from build123d import *

# Parameters (mm, degrees)
F0_W     = 28.575
F0_H     = 52.07
F1_DEPTH = 50.8
F2_R     = 11.1252
F3_DEPTH = 50.801
F4_R     = 1.5875
F5_DEPTH = 25.4


with BuildPart() as f1:
    # F0 (on Front) → F1 (new body)
    with BuildSketch(Plane.XZ):
        Rectangle(F0_W, F0_H)
    extrude(amount=F1_DEPTH)

    # F2 (on face) → F3 (cut, through all)
    with BuildSketch(Plane.XZ.offset(50.8)):
        with Locations((0, 11.641667)):
            Circle(F2_R)
        with Locations((0, -11.641667)):
            Circle(F2_R)
    extrude(amount=-F3_DEPTH, mode=Mode.SUBTRACT)

    # F4 (on face) → F5 (cut)
    with BuildSketch(Plane.YZ.offset(14.2875)):
        with Locations((-19.05, 0)):
            Circle(F4_R)
    extrude(amount=-F5_DEPTH, mode=Mode.SUBTRACT)


solid = f1.part
Work out the finished part from the listing and answer in its coordinate system (mm). A direction names the side the tool comes from. Coordinates: 2 decimals unless noted, no trailing zeros. Loops run counter-clockwise (first coordinate to the right, second up) from the corner with the lowest first, then second, coordinate; pieces in that order, holes last. Notation, with made-up numbers: (-9, 5.5) -> (31, 5.5) arc R18 ccw to (31, 30.5) -> close; hole circle Ø6 at (-19, 65). An arc over 180 degrees is marked (long way). Answer as CSV lines item,"result".
1) For faces 4 (the face through (1.765, -17.536, 0.477)), 5 (the face through (5.981, -25.756, 21.022)), determine the directions among +Z, -Z, +X, -X, +Y, -Y from which every point of the face is accessible in a straight line to the end or side of a thin tool.
A:
face 4,"+X"
face 5,"+Y, -Y"
2) Straight lines are drawn through the part: probe 1 along Z at (x, y) = (0, -23) (3 decimals); probe 2 along Z at (x, y) = (3, -8) (3 decimals); probe 3 along X at (y, z) = (-11, -10.5). For each, find the intervals that lie inside material, in ascending order.
A:
probe 1,"z = -26.035 to -22.767, -0.516 to 0.516, 22.767 to 26.035"
probe 2,"z = -26.035 to -22.355, -0.929 to 0.929, 22.355 to 26.035"
probe 3,"x = -14.29 to -11.07, 11.07 to 14.29"
3) The part is cut by section B-B (z = -17). Give the vertices of the cut face in (x, y).
A:
outline,"(-14.29, -50.8) -> (-9.75, -50.8) -> (-9.75, 0) -> (-14.29, 0) -> close; (9.75, -50.8) -> (14.29, -50.8) -> (14.29, 0) -> (9.75, 0) -> close"
4) For a pull along Z with two mould halves and no side action, classify faces 1 (the face through (0, -25, -26.035)), 2 (the face through (0, 0, 0)), 3 (the face through (-11.112, -19, 0)) as released by +Z, released by -Z, zero draft, split by the parting line, or undercut.
A:
face 1,"released by -Z"
face 2,"zero draft"
face 3,"undercut"
5) The part is cut by section A-A (x = -7.25). State how many separate pieces and enclosed holes the cut face has, and give its area (3 significant figures).
A:
separate pieces,"3"
enclosed holes,"1"
area,"923 mm²"
6) The part is cut by section D-D (y = -44). Give the vertices of the cut face in (x, z) (1 decimal), and give its area (3 significant figures).
A:
outline,"(-14.3, -26) -> (14.3, -26) -> (14.3, 26) -> (-14.3, 26) -> close; hole circle Ø22.3 at (0, -11.6); hole circle Ø22.3 at (0, 11.6)"
area,"710 mm²"
